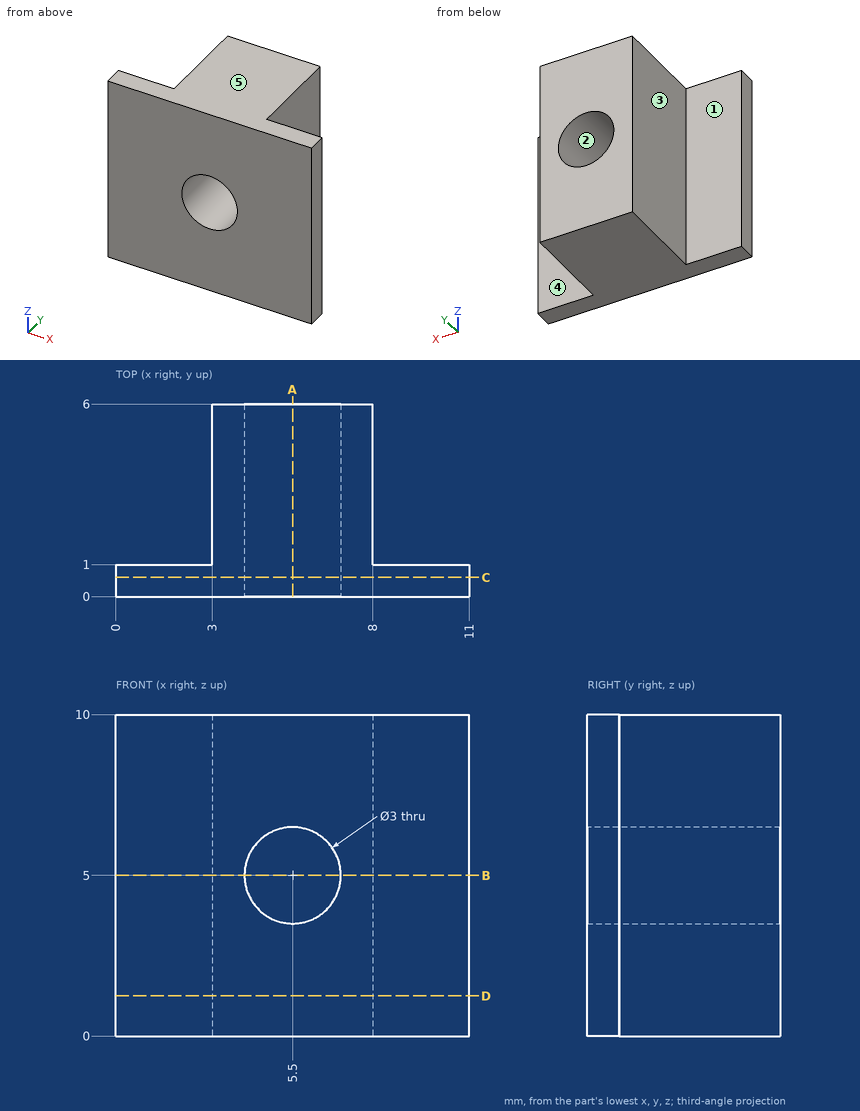
Study the drawing (mm; zero at the part's minimum x, y, z) and answer. A direction names the side the tool comes from. Give positions to 0.01 mm unless a question says otherwise; leave off trailing zeros. Order: outer loops, then holes, each group sorted by start corner. A loop starts at its lowest first (then second) coordinate and runs counter-clockwise, first axis right, second up.
1. Section A-A, the plane x = 5.5 is taken. Determine the outline of the cut face in (y, z), and give its area (3 significant figures).
Result sheet:
outline: (0, 0) - (6, 0) - (6, 3.5) - (0, 3.5) - close; (0, 6.5) - (6, 6.5) - (6, 10) - (0, 10) - close
area: 42.0 mm2
2. Straight lines are drawn through the part: L1, parallel to X at y = 3, z = 5; L2, parallel to X at y = 4.6, z = 9; L3, parallel to Y at x = 1.5, z = 0.5. For each, find the intervals that lie inside material, in ascending order.
Result sheet:
L1: x = 3 to 4, 7 to 8
L2: x = 3 to 8
L3: y = 0 to 1
3. Section D-D, the plane z = 1.25 is taken. Determine the outline of the cut face in (x, y), and give its area (3 significant figures).
Result sheet:
outline: (0, 0) - (11, 0) - (11, 1) - (8, 1) - (8, 6) - (3, 6) - (3, 1) - (0, 1) - close
area: 36.0 mm2
4. The mould has two halves that part along X. Classify the marked faces 1, 2 and 3: released by +X, released by -X, zero draft, split by the parting line, or undercut.
Result sheet:
face 1: zero draft
face 2: undercut
face 3: released by -X
5. For the marked faces 4 and 5, determine the directions among +Z, -Z, +X, -X, +Y, -Y from which every point of the face is accessible in a straight line to the end or side of a thin tool.
Result sheet:
face 4: +Z, -Z, +X, +Y
face 5: +Z, +X, -X, +Y, -Y
6. Each of these flat-tipped pins is pushed along its axis until it touches: P1, Ø2, axis at x = 3.5, z = 1.5, coming from the -Y side; P2, Ø2.5, axis at y = 3, z = 2.5, coming from the -X side; P3, Ø0.9, axis at x = 9, z = 5, coming from the +Y side; P4, Ø1.5, axis at y = 4.5, z = 4.5, coming from the +X side. Where does it stop, or does it pass through?
Result sheet:
P1: stops at y = 0
P2: stops at x = 3
P3: stops at y = 1
P4: stops at x = 8
7. Section B-B, the plane z = 5 is taken. Determine the outline of the cut face in (x, y).
Result sheet:
outline: (0, 0) - (4, 0) - (4, 6) - (3, 6) - (3, 1) - (0, 1) - close; (7, 0) - (11, 0) - (11, 1) - (8, 1) - (8, 6) - (7, 6) - close
8. Section C-C, the plane y = 0.6 is taken. Determine the outline of the cut face in (x, z), and give its area (3 significant figures).
Result sheet:
outline: (0, 0) - (11, 0) - (11, 10) - (0, 10) - close; hole circle Ø3 at (5.5, 5)
area: 103 mm2
